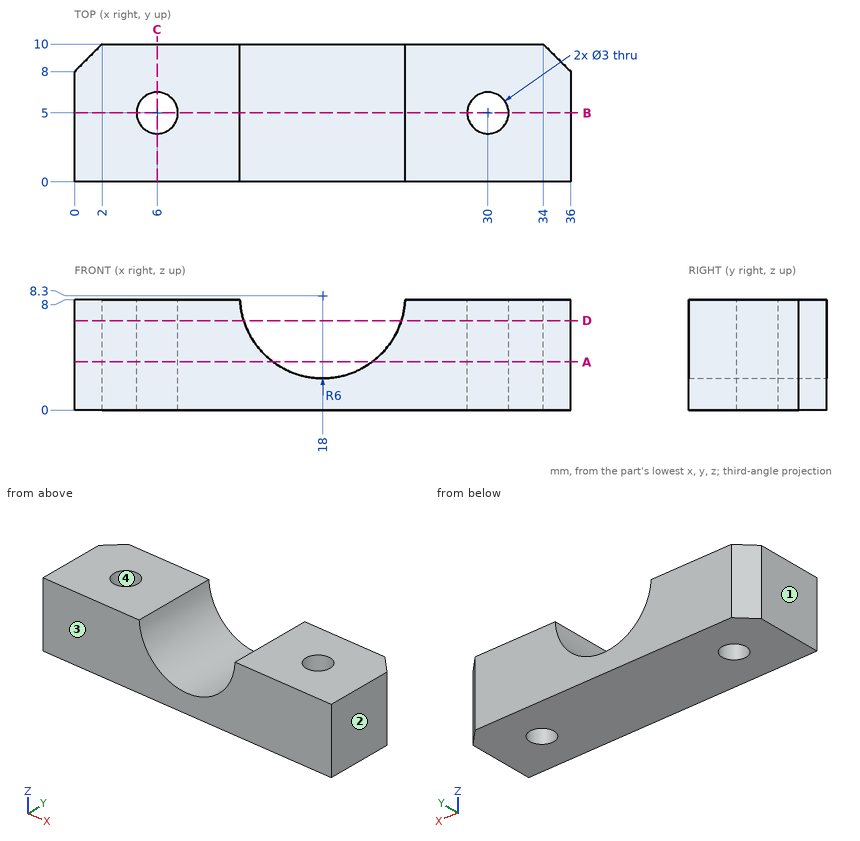
Print and shaded views of the part. All mm, measured from the part's lowest x, y and z. Round coordinates to 2 decimals unless told otherwise and drop trailing zeros. Order: outer loops, then holes, each group sorted by start corner. A loop starts at its lowest first (then second) coordinate and runs counter-clockwise, first axis right, second up.
Q1. Slice it at C-C (x = 6). Write the cut outline in (y, z), and give its area (3 significant figures).
Q2. Drop a flat-ended pin along its axis: pin 1 (1.5 mm diameter, centred on y = 9, z = 5, fed in from -X). Give the stop position or say it passes through.
Q3. Slice it at B-B (y = 5). Write the cut outline in (x, z), and give its area (3 significant figures).
Q4. Wall check: L1, parallel to Y at x = 6, z = 4.5; L2, parallel to X at y = 5, z = 3.25; L3, parallel to X at y = 5, z = 4.25. Give the ranges that are in metal, low to high.
Q5. Slice it at A-A (z = 3.5). Write the cut outline in (x, y), and give its area (3 significant figures).
Q6. Slice it at D-D (z = 6.5). Write the cut outline in (x, y).
Q7. Two-plate mould, pull along X, no slides. Class the marked faces 1, 2, 3 and 4: pulls with the +X half, pulls with the -X half, needs draft (parallel to the pull), parting line crosses it, or undercut.
Results below:
1. outline: (0, 0) - (3.5, 0) - (3.5, 8) - (0, 8) - close; (6.5, 0) - (10, 0) - (10, 8) - (6.5, 8) - close
1. area: 56.0 mm2
2. pin 1: stops at x = 0.25
3. outline: (0, 0) - (4.5, 0) - (4.5, 8) - (0, 8) - close; (7.5, 0) - (28.5, 0) - (28.5, 8) - (23.99, 8) arc R6 cw to (12.01, 8) - (7.5, 8) - close; (31.5, 0) - (36, 0) - (36, 8) - (31.5, 8) - close
3. area: 187 mm2
4. L1: y = 0 to 3.5, 6.5 to 10
4. L2: x = 0 to 4.5, 7.5 to 14.76, 21.24 to 28.5, 31.5 to 36
4. L3: x = 0 to 4.5, 7.5 to 13.57, 22.43 to 28.5, 31.5 to 36
5. outline: (0, 0) - (14.4, 0) - (14.4, 10) - (2, 10) - (0, 8) - close; (21.6, 0) - (36, 0) - (36, 8) - (34, 10) - (21.6, 10) - close; hole circle Ø3 at (6, 5); hole circle Ø3 at (30, 5)
5. area: 270 mm2
6. outline: (0, 0) - (12.28, 0) - (12.28, 10) - (2, 10) - (0, 8) - close; (23.72, 0) - (36, 0) - (36, 8) - (34, 10) - (23.72, 10) - close; hole circle Ø3 at (6, 5); hole circle Ø3 at (30, 5)
7. face 1: pulls with the -X half
7. face 2: pulls with the +X half
7. face 3: needs draft
7. face 4: undercut
